Read the model definition and answer for the solid it produces. Units are mm, in the model's axes. A direction names the side the tool comes from. Give positions to 0.01 mm unless a question says otherwise; leave off trailing zeros. Write each loop counter-clockwise with the first axis right and the second up, starting at its lowest first coordinate (ties: lowest second). Pieces come first, ordered by that corner, then holes. Notation, with made-up numbers: M -27.5,-23.75 L 7.5,-23.75 A4 ccw 7.5,-19.75 Z; hole C 40,60.25 d5. An arc over 180 degrees is marked long. Use a Markdown table: item, result. Add a question column.
Item 1: For faces 1 (the flat face through (5, 0, -15)), 2 (the flat face through (6, 14.4, 222)), 3 (the flat face through (5, 0, -30)), 4 (the flat face through (6, -14.4, -22)), determine the directions among +Z, -Z, +X, -X, +Y, -Y from which every point of the face is accessible in a straight line to the end or side of a thin tool.
Item 2: A cutting plane is placed at C-C on y = -2. Determine the outline of the cut face in (x, z), then the cut area to 3 significant figures.
Item 3: A cutting plane is placed at D-D on z = 7. Determine the outline of the cut face in (x, y), then the cut area to 3 significant figures.
Item 4: A cutting plane is placed at B-B on z = 219. Determine the outline of the cut face in (x, y).
Item 5: The mould has two halves that part along Z. Classify faces 5 (the flat face through (5, 0, 230)), 6 (the flat face through (12, 1, -40)), 7 (the flat face through (10, 1, 102)), 8 (the flat face through (12, -50, 102)): pulls with the +Z half, pulls with the -Z half, needs draft (parallel to the pull), parting line crosses it, or undercut.
Item 6: A cutting plane is placed at A-A on x = 7.75. Determine the outline of the cut face in (y, z), then the cut area to 3 significant figures.
Item 7: Consider probe 1 along Z at (x, y) = (2.25, -9); probe 2 along X at (y, z) = (6.5, 48). Determine where each line is inside the solid, lowest interval first. Write a range as [from, to].
Item 8: Given P1, Ø3, axis at x = 5, y = -2, coming from the -Z side; P2, Ø4.5, axis at x = 5, z = 220, coming from the -Y side; P3, Ø0.6, axis at x = 1, z = -24.5, coming from the +Y side, each flat-ended and moving along its own axis, determine where each tip first touches the part or whether it passes through.
from build123d import *

# Parameters (mm, degrees)
F1_START      = -15
F1_DEPTH      = 15
F2_DEPTH      = 240
F2_DEPTH_BACK = 40
F3_START      = 215
F3_DEPTH      = 15


with BuildPart() as f1:
    # F0 (on Top) → F1 (new body)
    with BuildSketch(Plane.XY.offset(F1_START)):
        Polygon((0, 17.4), (0, 0), (0, -17.4), (1.25, -17.4), (1.25, -14.4), (10, -14.4), (10, 14.4), (1.25, 14.4), (1.25, 17.4), align=None)
    extrude(amount=-F1_DEPTH)

    # F0 (on Top) → F2 (join, two sides)
    with BuildSketch(Plane.XY) as f2_sk:
        Polygon((10, 50), (10, 14.4), (10, -14.4), (10, -50), (15, -50), (15, 0), (15, 50), align=None)
    extrude(amount=F2_DEPTH)
    extrude(f2_sk.sketch, amount=-F2_DEPTH_BACK)

    # F0 (on Top) → F3 (join)
    with BuildSketch(Plane.XY.offset(F3_START)):
        Polygon((0, 17.4), (0, 0), (0, -17.4), (1.25, -17.4), (1.25, -14.4), (10, -14.4), (10, 14.4), (1.25, 14.4), (1.25, 17.4), align=None)
    extrude(amount=F3_DEPTH)


solid = f1.part
Filled in:
| question | item | result |
|---|---|---|
| 1 | face 1 | -X, +Y, -Y |
| 1 | face 2 | +Z, -Z, +Y |
| 1 | face 3 | -Z, -X, +Y, -Y |
| 1 | face 4 | +Z, -Z, -Y |
| 2 | outline | M 0,-30 L 10,-30 L 10,-40 L 15,-40 L 15,240 L 10,240 L 10,230 L 0,230 L 0,215 L 10,215 L 10,-15 L 0,-15 Z |
| 2 | area | 1,700 mm² |
| 3 | outline | M 10,-50 L 15,-50 L 15,50 L 10,50 Z |
| 3 | area | 500 mm² |
| 4 | outline | M 0,-17.4 L 1.25,-17.4 L 1.25,-14.4 L 10,-14.4 L 10,-50 L 15,-50 L 15,50 L 10,50 L 10,14.4 L 1.25,14.4 L 1.25,17.4 L 0,17.4 Z |
| 5 | face 5 | pulls with the +Z half |
| 5 | face 6 | pulls with the -Z half |
| 5 | face 7 | undercut |
| 5 | face 8 | needs draft |
| 6 | outline | M -14.4,-30 L 14.4,-30 L 14.4,-15 L -14.4,-15 Z; M -14.4,215 L 14.4,215 L 14.4,230 L -14.4,230 Z |
| 6 | area | 864 mm² |
| 7 | probe 1 | [-30, -15], [215, 230] |
| 7 | probe 2 | [10, 15] |
| 8 | P1 | z = -30 |
| 8 | P2 | y = -14.4 |
| 8 | P3 | y = 17.4 |
